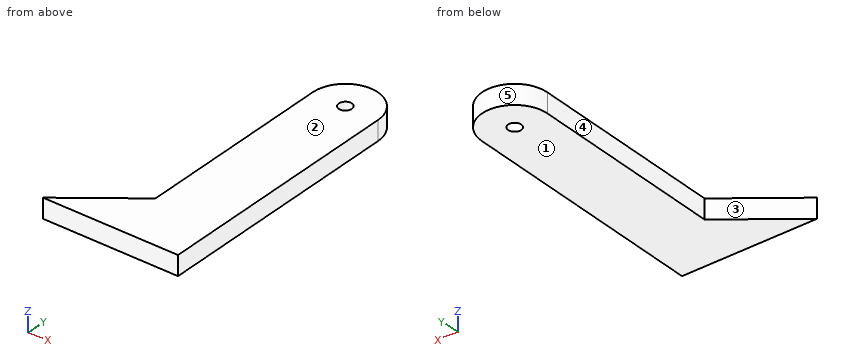
from build123d import *

# Parameters (mm, degrees)
SKETCH_1_R      = 1
EXTRUDE_1_DEPTH = 3
EXTRUDE_2_DEPTH = 3


with BuildPart() as part:
    # 草图1 → 凸台-拉伸1 (new body)
    with BuildSketch(Plane.XY):
        with BuildLine():
            Line((-5, 0), (-5, -30.357146931))
            Line((-5, -30.357146931), (5, -30.357146931))
            Line((5, -30.357146931), (5, 0))
            ThreePointArc((5, 0), (0, 5), (-5, 0))
        make_face()
        Circle(SKETCH_1_R, mode=Mode.SUBTRACT)
    extrude(amount=EXTRUDE_1_DEPTH)

    # 草图2 → 凸台-拉伸2 (add)
    with BuildSketch(Plane.XY.offset(3)):
        Polygon((-15.678069464, -38.606948739), (5, -38.606948739), (5, -35.668972407), (5, -30.357146931), (-5, -30.357146931), align=None)
    extrude(amount=-EXTRUDE_2_DEPTH)


solid = part.part
Verification items for the finished model (mm, model axes). Face numbers are marked on the shaded views. A direction names the side the tool comes from. Give positions to 0.01 mm unless a question says otherwise; leave off trailing zeros. Write each loop counter-clockwise with the first axis right and the second up, starting at its lowest first coordinate (ties: lowest second). Pieces come first, ordered by that corner, then holes.
(1) Gauge pin test, flat end, axial feed: pin 1 (1 mm diameter, centred on y = -21.5, z = 2.5, fed in from -X). Record the tip position at first contact, or that the pin passes through.
(2) Cross-section at C-C (y = -23.5). Enter the section's corners in (x, z).
(3) Cross-section at A-A (x = 0). Enter the section's corners in (y, z), plus the area to 3 significant figures.
(4) Material ranges on line 1 (Y direction, x = 0, z = 1.05); line 2 (X direction, y = -1.5, z = 1.9); line 3 (Y direction, x = -9, z = 1.15), recorded low to high.
(5) Access from +Z, -Z, +X, -X, +Y, -Y to the whole of each face (thin tool, end or side, straight path). Record for the marked faces 4 and 5.
(6) Cross-section at B-B (z = 1.45). Enter the section's corners in (x, y), plus the area to 3 significant figures.
(7) Mould release check, pull along Z, two halves, no side actions. Record for the marked faces 1, 2 and 3: +Z half, -Z half, draft (parallel to the pull), parting line (faces both ways), or undercut.
(8) Cross-section at D-D (x = -11). Enter the section's corners in (y, z).
Worked out:
1. pin 1: stops at x = -5
2. outline: (-5, 0) - (5, 0) - (5, 3) - (-5, 3) - close
3. outline: (-38.61, 0) - (-1, 0) - (-1, 3) - (-38.61, 3) - close; (1, 0) - (5, 0) - (5, 3) - (1, 3) - close
3. area: 125 mm2
4. line 1: y = -38.61 to -1, 1 to 5
4. line 2: x = -5 to 5
4. line 3: y = -38.61 to -33.45
5. face 4: +Z, -Z, -X, +Y
5. face 5: +Z, -Z, +Y
6. outline: (-15.68, -38.61) - (5, -38.61) - (5, 0) arc R5 ccw to (-5, 0) - (-5, -30.36) - close; hole circle Ø2 at (0, 0)
6. area: 466 mm2
7. face 1: -Z half
7. face 2: +Z half
7. face 3: draft
8. outline: (-38.61, 0) - (-34.99, 0) - (-34.99, 3) - (-38.61, 3) - close
